Work out the finished part from the listing and answer in its coordinate system (mm). Face numbers are marked on the shaded views. A direction names the side the tool comes from. Round coordinates to 2 decimals unless told otherwise and drop trailing zeros. Write each loop counter-clockwise with the first axis right and the second up, starting at its lowest first coordinate (ties: lowest second). Pieces come first, ordered by that corner, then holes.
1. Find section C-C (z = 1.25). Write down the section's boundary in (x, y) (3 decimals), and give its area (3 significant figures).
2. Straight lines are drawn through the part: probe 1 along X at (y, z) = (-15.5, 7.5) (3 decimals); probe 2 along X at (y, z) = (9, 8.75) (3 decimals); probe 3 along X at (y, z) = (33, 14). For each, find the intervals that lie inside material, in ascending order.
3. Find section D-D (y = -7). Write down the section's boundary in (x, z) (1 decimal), and give its area (3 significant figures).
4. A tool of negligible diameter and unlimited length cuts with its end or side. For the marked faces 4, 5, 6, 7 and 8, from which of +Z, -Z, +X, -X, +Y, -Y can it reach the whole face along a straight path? Write none if from no direction.
5. Find section B-B (z = 6.75). Write down the section's boundary in (x, y) (3 decimals).
6. Flat-ended cylindrical pins translate along their axes: pin 1 Ø7 at (x, z) = (-39.69, 7.94) entering from -Y; pin 2 Ø6 at (x, z) = (-31, 5) entering from +Y; pin 3 Ø4 at (x, z) = (-11.5, 6.5) entering from +Y; pin 4 Ø6 at (x, z) = (39.69, 7.94) entering from -Y. Find the tip coordinate at first contact, or state that the pin passes through.
7. Find section A-A (y = 36.5). Write down the section's boundary in (x, z) (3 decimals).
8. Determine the mould class of the marked faces 1, 2 and 3 for opening direction X: pulls with the +X half, pulls with the -X half, needs draft (parallel to the pull), parting line crosses it, or undercut.
```python
from build123d import *

# Parameters (mm, degrees)
BOSS_EXTRUDE1_DEPTH                = 15.875
F_1_4_CLEARANCE_HOLE1_D            = 6.7564
F_1_16_0_0625_DIAMETER_HOLE1_D     = 11.43
F_1_16_0_0625_DIAMETER_HOLE1_DEPTH = 33.3756
FILLET1_R                          = 7.62


with BuildPart() as part:
    # Sketch1 → Boss-Extrude1 (new body)
    with BuildSketch(Plane.XY):
        Polygon((31.75, 31.75), (-31.75, 31.75), (-31.75, 19.05), (-47.625, 19.05), (-47.625, -31.75), (47.625, -31.75), (47.625, 19.05), (31.75, 19.05), align=None)
        Polygon((-31.75, 40.162272173), (-31.75, 31.75), (31.75, 31.75), (31.75, 40.162272173), (19.119534727, 38.078833297), (0, 34.925), (-19.119537229, 38.07883371), align=None)
    extrude(amount=BOSS_EXTRUDE1_DEPTH)

    # 1/4 Clearance Hole1 (through all)
    with Locations(Plane(origin=(0, 19.05, 0), x_dir=(-1, 0, 0), z_dir=(0, 1, 0))):
        with Locations((39.6875, 7.9375), (-39.6875, 7.9375)):
            Hole(F_1_4_CLEARANCE_HOLE1_D / 2)

    # 1/16 (0.0625) Diameter Hole1
    with Locations(Plane.XZ.offset(31.75)):
        with Locations((39.6875, 7.9375), (-39.6875, 7.9375)):
            Hole(F_1_16_0_0625_DIAMETER_HOLE1_D / 2, depth=F_1_16_0_0625_DIAMETER_HOLE1_DEPTH)

    # Fillet1
    fillet1_edges = [part.edges().sort_by_distance(p)[0] for p in [
        (0, 34.925, 7.9375),
    ]]
    fillet(fillet1_edges, radius=FILLET1_R)


solid = part.part
```
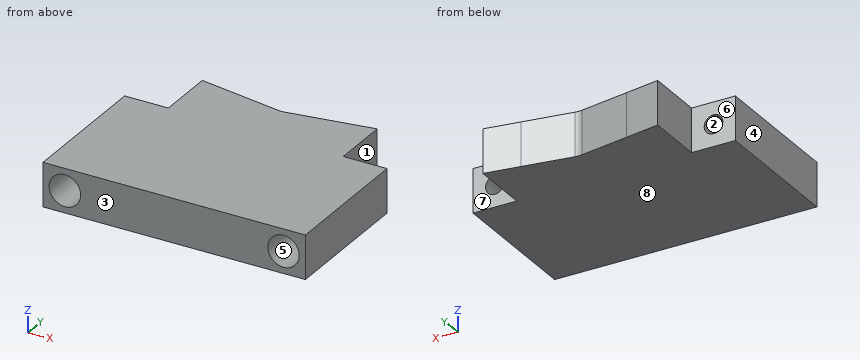
Worked answers:
1. outline: (-47.625, -31.75) - (47.625, -31.75) - (47.625, 19.05) - (31.75, 19.05) - (31.75, 40.162) - (1.24, 35.13) arc R7.62 cw to (-1.24, 35.13) - (-31.75, 40.162) - (-31.75, 19.05) - (-47.625, 19.05) - close
1. area: 6,010 mm2
2. probe 1: x = -47.625 to -45.386, -33.989 to 33.989, 45.386 to 47.625
2. probe 2: x = -47.625 to -42.967, -36.408 to 36.408, 42.967 to 47.625
2. probe 3: x = -31.75 to 31.75
3. outline: (-47.6, 0) - (47.6, 0) - (47.6, 15.9) - (-47.6, 15.9) - close; hole circle Ø11.4 at (-39.7, 7.9); hole circle Ø11.4 at (39.7, 7.9)
3. area: 1,310 mm2
4. face 4: +Z, -Z, -X, +Y, -Y
4. face 5: -Y
4. face 6: +Z, -Z, -X, +Y
4. face 7: +Z, -Z, +X, +Y
4. face 8: -Z, +X, -X, +Y, -Y
5. outline: (-47.625, -31.75) - (-45.278, -31.75) - (-45.278, 1.626) - (-42.85, 1.626) - (-42.85, 19.05) - (-47.625, 19.05) - close; (-36.525, 1.626) - (-34.097, 1.626) - (-34.097, -31.75) - (34.097, -31.75) - (34.097, 1.626) - (36.525, 1.626) - (36.525, 19.05) - (31.75, 19.05) - (31.75, 40.162) - (1.24, 35.13) arc R7.62 cw to (-1.24, 35.13) - (-31.75, 40.162) - (-31.75, 19.05) - (-36.525, 19.05) - close; (42.85, 1.626) - (45.278, 1.626) - (45.278, -31.75) - (47.625, -31.75) - (47.625, 19.05) - (42.85, 19.05) - close
6. pin 1: stops at y = 1.63
6. pin 2: stops at y = 40.16
6. pin 3: stops at y = 37.15
6. pin 4: passes through
7. outline: (-31.75, 0) - (-9.548, 0) - (-9.548, 15.875) - (-31.75, 15.875) - close; (9.548, 0) - (31.75, 0) - (31.75, 15.875) - (9.548, 15.875) - close
8. face 1: pulls with the +X half
8. face 2: undercut
8. face 3: needs draft
